The listing builds one solid part. Answer for the finished solid, in the listing's coordinates (mm). Coordinates: 2 decimals unless noted, no trailing zeros. Order: outer loops, then holes, each group sorted by start corner. A loop starts at its lowest first (then second) coordinate and runs counter-clockwise, first axis right, second up. Notation, with made-up numbers: (-13.5, 34.5) -> (32.5, 34.5) arc R22 cw to (32.5, 62.5) -> close; hole circle Ø7 at (40, -26). An arc over 180 degrees is marked (long way). Return JSON: item names as keys, results as strings.
from build123d import *

# Parameters (mm, degrees)
SKETCH1_W           = 26.7
SKETCH1_H           = 14.9
BOSS_EXTRUDE1_DEPTH = 1
FILLET1_R           = 0.1
SKETCH2_W           = 21.744
SKETCH2_H           = 10.864
CUT_EXTRUDE1_DEPTH  = 0.1


with BuildPart() as part:
    # Sketch1 → Boss-Extrude1 (new body)
    with BuildSketch(Plane.XY):
        Rectangle(SKETCH1_W, SKETCH1_H)
    extrude(amount=BOSS_EXTRUDE1_DEPTH)

    # Fillet1
    fillet1_edges = [part.edges().sort_by_distance(p)[0] for p in [
        (13.35, -7.45, 0.5),
        (-13.35, -7.45, 0.5),
        (-13.35, 7.45, 0.5),
        (13.35, 7.45, 0.5),
    ]]
    fillet(fillet1_edges, radius=FILLET1_R)

    # Sketch2 → Cut-Extrude1 (cut)
    with BuildSketch(Plane(origin=(0, 0, 0), x_dir=(-1, 0, 0), z_dir=(0, 0, -1))):
        with Locations((0, -0.082)):
            Rectangle(SKETCH2_W, SKETCH2_H)
    extrude(amount=-CUT_EXTRUDE1_DEPTH, mode=Mode.SUBTRACT)


solid = part.part
1. This flat-tipped pin is pushed along its axis until it touches: pin 1 Ø1.5 at (x, y) = (-5.5, -3.5) entering from -Z. Where does it stop, or does it pass through?
Answer block:
{"pin 1": "stops at z = 0.1"}
2. The part is cut by section A-A on x = 6. Give the vertices of the cut face in (y, z), and give its area (3 significant figures).
Answer block:
{"outline": "(-7.45, 0) -> (-5.51, 0) -> (-5.51, 0.1) -> (5.35, 0.1) -> (5.35, 0) -> (7.45, 0) -> (7.45, 1) -> (-7.45, 1) -> close", "area": "13.8 mm2"}
3. Consider line 1 (Z direction, x = -8.5, y = 5); line 2 (Y direction, x = -3.25, z = 0.05). Determine where each line is inside the solid, lowest interval first. Write a range as from..to.
Answer block:
{"line 1": "z = 0.1..1", "line 2": "y = -7.45..-5.51, 5.35..7.45"}
4. The part is cut by section B-B on y = 2.75. Give the vertices of the cut face in (x, z).
Answer block:
{"outline": "(-13.35, 0) -> (-10.87, 0) -> (-10.87, 0.1) -> (10.87, 0.1) -> (10.87, 0) -> (13.35, 0) -> (13.35, 1) -> (-13.35, 1) -> close"}
5. Determine the mould class of faces 1 (the face through (0, 0, 0.1)), 2 (the face through (-13.35, -0.1, 0.5)), 3 (the face through (-0.2, 7.45, 0.5)), 4 (the face through (13.35, -0.1, 0.5)) for opening direction X: pulls with the +X half, pulls with the -X half, needs draft (parallel to the pull), parting line crosses it, or undercut.
Answer block:
{"face 1": "undercut", "face 2": "pulls with the -X half", "face 3": "needs draft", "face 4": "pulls with the +X half"}
